from build123d import *

# Parameters (mm, degrees)
F0_R     = 10
F0_R_2   = 5
F1_DEPTH = 16
F0_R_3   = 12
F2_DEPTH = 11
F3_DEPTH = 10
F4_DEPTH = 10
F5_DEPTH = 11


with BuildPart() as f1:
    # F0 (on Top) → F1 (new body)
    with BuildSketch(Plane.XY):
        Polygon((4.8361202547, -10.664289076), (11.3529485972, -2.8680444149), (9.320775088, 7.0878961882), (0.2698678284, 11.7065063948), (-8.9842554103, 7.5098785169), (-11.4730510796, -2.3418410578), (-5.3224052784, -10.4301065511), align=None)
        Circle(F0_R, mode=Mode.SUBTRACT)
        Circle(F0_R)
        Polygon((9.1977509421, -2.0993266316), (4.0933842599, -8.5), (-4.0933842599, -8.5), (-9.1977509421, -2.0993266316), (-7.376023565, 5.8821825089), (0, 9.4342882455), (7.376023565, 5.8821825089), align=None, mode=Mode.SUBTRACT)
        Polygon((-4.0933842599, -8.5), (4.0933842599, -8.5), (9.1977509421, -2.0993266316), (7.376023565, 5.8821825089), (0, 9.4342882455), (-7.376023565, 5.8821825089), (-9.1977509421, -2.0993266316), align=None)
        Circle(F0_R_2, mode=Mode.SUBTRACT)
    extrude(amount=F1_DEPTH)

    # F0 (on Top) → F2 (join)
    with BuildSketch(Plane.XY):
        Circle(F0_R_3)
        Polygon((9.320775088, 7.0878961882), (11.3529485972, -2.8680444149), (4.8361202547, -10.664289076), (-5.3224052784, -10.4301065511), (-11.4730510796, -2.3418410578), (-8.9842554103, 7.5098785169), (0.2698678284, 11.7065063948), align=None, mode=Mode.SUBTRACT)
    extrude(amount=F2_DEPTH)

    # F0 (on Top) → F3 (cut)
    with BuildSketch(Plane.XY):
        Circle(F0_R_3)
        Polygon((9.320775088, 7.0878961882), (11.3529485972, -2.8680444149), (4.8361202547, -10.664289076), (-5.3224052784, -10.4301065511), (-11.4730510796, -2.3418410578), (-8.9842554103, 7.5098785169), (0.2698678284, 11.7065063948), align=None, mode=Mode.SUBTRACT)
    extrude(amount=F3_DEPTH, mode=Mode.SUBTRACT)

    # F0 (on Top) → F4 (cut)
    with BuildSketch(Plane.XY):
        Polygon((4.8361202547, -10.664289076), (11.3529485972, -2.8680444149), (9.320775088, 7.0878961882), (0.2698678284, 11.7065063948), (-8.9842554103, 7.5098785169), (-11.4730510796, -2.3418410578), (-5.3224052784, -10.4301065511), align=None)
        Circle(F0_R, mode=Mode.SUBTRACT)
    extrude(amount=F4_DEPTH, mode=Mode.SUBTRACT)

    # F0 (on Top) → F5 (join)
    with BuildSketch(Plane.XY):
        Polygon((-4.0933842599, -8.5), (4.0933842599, -8.5), (9.1977509421, -2.0993266316), (7.376023565, 5.8821825089), (0, 9.4342882455), (-7.376023565, 5.8821825089), (-9.1977509421, -2.0993266316), align=None)
        Circle(F0_R_2, mode=Mode.SUBTRACT)
    extrude(amount=-F5_DEPTH)


solid = f1.part
Work out the finished part from the listing and answer in its coordinate system (mm). A direction names the side the tool comes from. Coordinates: 2 decimals unless noted, no trailing zeros. Order: outer loops, then holes, each group sorted by start corner. A loop starts at its lowest first (then second) coordinate and runs counter-clockwise, first axis right, second up. Notation, with made-up numbers: (55.25, 30) - (81.25, 30) arc R17 ccw to (81.25, 40) - close; hole circle Ø10 at (46.5, 43). An arc over 180 degrees is marked (long way). Put each result on its own line as item: value. Start each with the question number.
1) Find section B-B (x = -3.25). Give the vertices of the cut face in (y, z), plus the area to 3 significant figures.
2) Find section C-C (y = 2.75). Give the vertices of the cut face in (x, z).
3) Find the intervals of material crossed by line 1 (Y direction, x = 0, z = -7); line 2 (Y direction, x = 0, z = 8.5); line 3 (Z direction, x = -4, y = 10), in increasing order. Write a range as from..to.
4) Find section D-D (z = -5.25). Give the vertices of the cut face in (x, y).
5) For faces 1 (the flat face through (-10.2, 2.7, 13.5)), 2 (the flat face through (-8.274, 1.947, -5.423)), 3 (the flat face through (-5, 9, 10)), 4 (the flat face through (-8.44, -6.33, 13.46)), 5 (the flat face through (8.3, 1.84, -5.42)), determine the directions among +Z, -Z, +X, -X, +Y, -Y from which every point of the face is accessible in a straight line to the end or side of a thin tool.
6) Flat-ended cylindrical pins translate along their axes: pin 1 (8 mm diameter, centred on x = -1, z = -5.5, fed in from +Y); pin 2 (4 mm diameter, centred on x = -3, z = -6, fed in from +Y); pin 3 (6 mm diameter, centred on x = 0, y = 0, fed in from +Z); pin 4 (8 mm diameter, centred on x = 9, z = -7, fed in from -Y). Find the tip coordinate at first contact, or state that the pin passes through.
7) Find section A-A (z = 12). Give the vertices of the cut face in (x, y), plus the area to 3 significant figures.
Results list:
1. outline: (-11.55, 10) - (-9.46, 10) - (-9.46, 0) - (-8.5, 0) - (-8.5, -11) - (-3.8, -11) - (-3.8, 16) - (-10.48, 16) - (-10.48, 11) - (-11.55, 11) - close; (3.8, -11) - (7.87, -11) - (7.87, 0) - (9.46, 0) - (9.46, 10) - (11.55, 10) - (11.55, 11) - (10.11, 11) - (10.11, 16) - (3.8, 16) - close
1. area: 290 mm^2
2. outline: (-11.68, 10) - (-9.61, 10) - (-9.61, 0) - (-8.09, 0) - (-8.09, -11) - (-4.18, -11) - (-4.18, 16) - (-10.19, 16) - (-10.19, 11) - (-11.68, 11) - close; (4.18, -11) - (8.09, -11) - (8.09, 0) - (9.61, 0) - (9.61, 10) - (11.68, 10) - (11.68, 11) - (10.21, 11) - (10.21, 16) - (4.18, 16) - close
3. line 1: y = -8.5..-5, 5..9.43
3. line 2: y = -10..-5, 5..10
3. line 3: z = 10..11
4. outline: (-9.2, -2.1) - (-4.09, -8.5) - (4.09, -8.5) - (9.2, -2.1) - (7.38, 5.88) - (0, 9.43) - (-7.38, 5.88) - close; hole circle Ø10 at (0, 0)
5. face 1: +Z, -X, +Y
5. face 2: -Z, -X, +Y
5. face 3: -Z
5. face 4: +Z, -X, -Y
5. face 5: -Z, +X, +Y
6. pin 1: stops at y = 9.43
6. pin 2: stops at y = 8.95
6. pin 3: passes through
6. pin 4: stops at y = -7.36
7. outline: (-11.47, -2.34) - (-5.32, -10.43) - (4.84, -10.66) - (11.35, -2.87) - (9.32, 7.09) - (0.27, 11.71) - (-8.98, 7.51) - close; hole circle Ø10 at (0, 0)
7. area: 297 mm^2
